Source: CAD feature listing. Evaluate the final solid. Frame: model axes, mm. Round coordinates to 2 decimals unless told otherwise and drop trailing zeros. Order: outer loops, then holes, each group sorted by start corner. A loop starts at its lowest first (then second) coordinate and runs counter-clockwise, first axis right, second up.
```python
from build123d import *

# Parameters (mm, degrees)
F0_W     = 400
F0_H     = 1600
F1_DEPTH = 12.5
F2_SIZE  = 24.99999


# Not quite as in the source:
# - a fillet or chamfer is up to 0.001 mm smaller than in the source, because OpenCascade refuses the exact size


with BuildPart() as f1:
    # F0 (on Top) → F1 (new body, symmetric)
    with BuildSketch(Plane.XY):
        Rectangle(F0_W, F0_H)
    extrude(amount=F1_DEPTH, both=True)

    # F2 (size 25 in the source; OpenCascade refuses exactly that, so slightly less here)
    f2_edges = [f1.edges().sort_by_distance(p)[0] for p in [
        (0, -800, -12.5),
        (0, 800, -12.5),
        (200, 0, -12.5),
    ]]
    chamfer(f2_edges, length=F2_SIZE)


solid = f1.part
```
1. First-contact query: pin 1 (2 mm diameter, centred on y = -338.5, z = -1, fed in from +X); pin 2 (12 mm diameter, centred on x = 105, z = -1.5, fed in from +Y); pin 3 (4 mm diameter, centred on x = 96.5, z = 1, fed in from -Y). Flat tips, straight axial feed; report the tip coordinate or a pass-through.
2. Section C-C on z = -3. Return loops of the section in (x, y), plus the area to 3 significant figures.
3. Line query: line 1 along Y through (x, z) = (-38.5, -8.25); line 2 along Y through (x, z) = (-118.5, -10.25); line 3 along X through (y, z) = (-690, -4.25). Output: solid intervals per line, ascending.
Result:
1. pin 1: stops at x = 187.5
1. pin 2: stops at y = 792
1. pin 3: stops at y = -790.5
2. outline: (-200, -784.5) - (184.5, -784.5) - (184.5, 784.5) - (-200, 784.5) - close
2. area: 603,000 mm2
3. line 1: y = -779.25 to 779.25
3. line 2: y = -777.25 to 777.25
3. line 3: x = -200 to 183.25
